Could you check a few things on this model? Use its own coordinates, in mm. Round coordinates to 2 decimals unless told otherwise and drop trailing zeros. Write each loop counter-clockwise with the first axis right and the second up, starting at its lowest first coordinate (ties: lowest second). Pieces come first, ordered by that corner, then holes. Notation, with made-up numbers: (-32, 73) -> (24, 73) arc R21 ccw to (24, 81) -> close; hole circle Ø5 at (74.25, 36). An arc over 180 degrees is marked (long way). Answer in a Markdown table with one row per item. Add a question column.
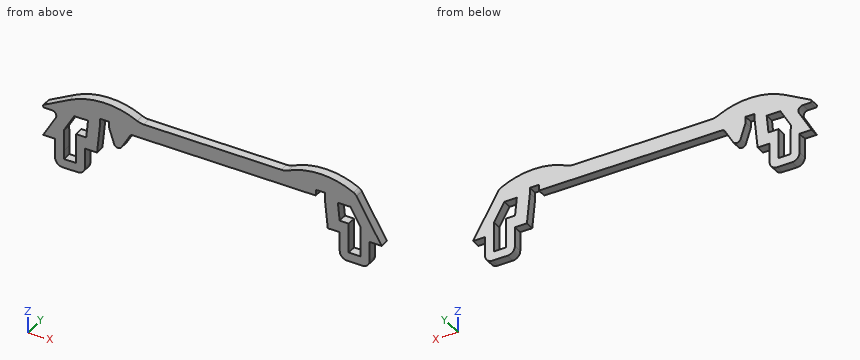
```python
from build123d import *

# Parameters (mm, degrees)
BOSS_EXTRUDE1_DEPTH = 3
FILLET2_R           = 2.5
FILLET3_R           = 1
FILLET5_R           = 2.5
FILLET6_R           = 5


with BuildPart() as part:
    # Sketch1 → Boss-Extrude1 (new body)
    with BuildSketch(Plane(origin=(0, 0, 0), x_dir=(1, 0, 0), z_dir=(0, 1, 0))):
        with BuildLine():
            Line((-62.418566214, -47.137504987), (-58.418566214, -47.137504987))
            Line((-58.418566214, -47.137504987), (-58.418566214, -38.137504987))
            Line((-58.418566214, -38.137504987), (-48.418566214, -38.137504987))
            Line((-48.418566214, -38.137504987), (-48.418566214, -47.137504987))
            Line((-48.418566214, -47.137504987), (-44.418566214, -47.137504987))
            Line((-44.418566214, -47.137504987), (-43.418817081, -57.134996312))
            Line((-43.418817081, -57.134996312), (-43.418817081, -59.137504987))
            Line((-43.418817081, -59.137504987), (-40.418817081, -59.137504987))
            Line((-40.418817081, -59.137504987), (-40.418817081, -57.137504987))
            Line((-40.418817081, -57.137504987), (-38.722684913, -52.023499684))
            ThreePointArc((-38.722684913, -52.023499684), (-37.561438496, -51.091888176), (-36.235977812, -51.769787298))
            Line((-36.235977812, -51.769787298), (-33.13692456, -57.137504987))
            Line((-33.13692456, -57.137504987), (28.581433786, -57.137504987))
            Line((28.581433786, -57.137504987), (28.581433786, -59.137504987))
            Line((28.581433786, -59.137504987), (31.581433786, -59.137504987))
            Line((31.581433786, -59.137504987), (31.581433786, -57.187643384))
            Line((31.581433786, -57.187643384), (32.581433786, -47.190177149))
            Line((32.581433786, -47.190177149), (36.581433786, -47.190177149))
            Line((36.581433786, -47.190177149), (36.581433786, -38.190177149))
            Line((36.581433786, -38.190177149), (46.581433786, -38.190177149))
            Line((46.581433786, -38.190177149), (46.581433786, -47.190177149))
            Line((46.581433786, -47.190177149), (50.581433786, -47.190177149))
            Line((50.581433786, -47.190177149), (41.830582941, -62.137504987))
            ThreePointArc((41.830582941, -62.137504987), (30.081433786, -65.137504987), (18.332284631, -62.137504987))
            Line((18.332284631, -62.137504987), (-30.079321987, -62.137504987))
            ThreePointArc((-30.079321987, -62.137504987), (-41.918817081, -65.137504987), (-53.758312176, -62.137504987))
            Line((-53.758312176, -62.137504987), (-62.202371167, -57.589552191))
            ThreePointArc((-62.202371167, -57.589552191), (-62.450096964, -57.027082233), (-61.965274707, -56.649341709))
            Line((-61.965274707, -56.649341709), (-59.524980934, -56.649341709))
            ThreePointArc((-59.524980934, -56.649341709), (-58.225942828, -55.899341709), (-58.225942828, -54.399341709))
            Line((-58.225942828, -54.399341709), (-62.418566214, -47.137504987))
        make_face()
        Polygon((36.547763078, -51.190177149), (39.581433786, -51.190177149), (39.581433786, -44.190177149), (39.581433786, -41.190177149), (43.581433786, -41.190177149), (43.581433786, -44.22970007), (43.581433786, -51.22970007), (40.093380681, -57.187643384), (35.947864455, -57.187643384), align=None, mode=Mode.SUBTRACT)
        Polygon((-55.418566214, -41.137504987), (-51.418566214, -41.137504987), (-51.418566214, -44.137504987), (-51.418566214, -51.137504987), (-48.038516462, -51.137504987), (-47.438516462, -57.137504987), (-52.026261368, -57.137504987), (-55.490362984, -51.137504987), (-55.418566214, -44.137873195), align=None, mode=Mode.SUBTRACT)
    extrude(amount=BOSS_EXTRUDE1_DEPTH)

    # Fillet2
    fillet2_edges = [part.edges().sort_by_distance(p)[0] for p in [
        (-58.418566214, 1.5, 38.137504987),
        (-48.418566214, 1.5, 38.137504987),
        (36.581433786, 1.5, 38.190177149),
        (46.581433786, 1.5, 38.190177149),
    ]]
    fillet(fillet2_edges, radius=FILLET2_R)

    # Fillet3
    fillet3_edges = [part.edges().sort_by_distance(p)[0] for p in [
        (-33.13692456, 1.5, 57.137504987),
    ]]
    fillet(fillet3_edges, radius=FILLET3_R)

    # Fillet5
    fillet5_edges = [part.edges().sort_by_distance(p)[0] for p in [
        (41.830582941, 1.5, 62.137504987),
        (-53.758312176, 1.5, 62.137504987),
    ]]
    fillet(fillet5_edges, radius=FILLET5_R)

    # Fillet6
    fillet6_edges = [part.edges().sort_by_distance(p)[0] for p in [
        (18.332284631, 1.5, 62.137504987),
        (-30.079321987, 1.5, 62.137504987),
    ]]
    fillet(fillet6_edges, radius=FILLET6_R)


solid = part.part
```
(1) Suppose I cut it at B-B, the plane y = 2.1. State how many separate pieces and enclosed holes the cut face has, then the cut area to 3 significant figures.
(2) Suppose I cut it at A-A, the plane z = 42.5. Please give me the cut outline in (x, y), then the cut area to 3 significant figures.
(3) I need wall thicknesses on L1, parallel to X at y = 1.95, z = 43.25; L2, parallel to X at y = 2.85, z = 56; L3, parallel to X at y = 0.5, z = 55.75. Which ranges of each line are inside material? Lowest first, please.
(4) Suppose I cut it at C-C, the plane z = 49.25. Please give me the cut outline in (x, y).
(5) For P1, Ø1.6, axis at y = 1, z = 58, coming from the +X side; P2, Ø1.5, axis at y = 1.5, z = 45, coming from the +X side; P3, Ø0.9, axis at x = 41.5, y = 1.5, coming from the +Z side, each with a flat end and sliding along its axis, tell me the tip position at first contact or that it passes through.
(6) Suppose I cut it at D-D, the plane x = 2.5. Please give me the cut outline in (y, z), then the cut area to 3 significant figures.
Response:
| question | item | result |
|---|---|---|
| 1 | separate pieces | 1 |
| 1 | enclosed holes | 2 |
| 1 | area | 959 mm² |
| 2 | outline | (-58.42, 0) -> (-55.42, 0) -> (-55.42, 3) -> (-58.42, 3) -> close; (-51.42, 0) -> (-48.42, 0) -> (-48.42, 3) -> (-51.42, 3) -> close; (36.58, 0) -> (39.58, 0) -> (39.58, 3) -> (36.58, 3) -> close; (43.58, 0) -> (46.58, 0) -> (46.58, 3) -> (43.58, 3) -> close |
| 2 | area | 36.0 mm² |
| 3 | L1 | -58.42 to -55.42, -51.42 to -48.42, 36.58 to 39.58, 43.58 to 46.58 |
| 3 | L2 | -58.29 to -52.68, -47.55 to -43.53, -40.04 to -33.79, 31.7 to 36.07, 40.79 to 45.42 |
| 3 | L3 | -58.15 to -52.83, -47.58 to -43.56, -39.96 to -33.94, 31.73 to 36.09, 40.94 to 45.57 |
| 4 | outline | (-61.2, 0) -> (-55.47, 0) -> (-55.47, 3) -> (-61.2, 3) -> close; (-51.42, 0) -> (-44.21, 0) -> (-44.21, 3) -> (-51.42, 3) -> close; (32.38, 0) -> (39.58, 0) -> (39.58, 3) -> (32.38, 3) -> close; (43.58, 0) -> (49.38, 0) -> (49.38, 3) -> (43.58, 3) -> close |
| 5 | P1 | x = 44.72 |
| 5 | P2 | x = 46.58 |
| 5 | P3 | z = 62.55 |
| 6 | outline | (0, 57.14) -> (3, 57.14) -> (3, 62.14) -> (0, 62.14) -> close |
| 6 | area | 15.0 mm² |
